Could you check a few things on this model? Use its own coordinates, in mm. A direction names the side the tool comes from. Coordinates: 2 decimals unless noted, no trailing zeros. Order: outer loops, then holes, each group sorted by start corner. A loop starts at its lowest first (then second) coordinate and runs counter-clockwise, first axis right, second up. Notation, with made-up numbers: (35, 1.25) - (41, 1.25) arc R16 cw to (41, 8.25) - close; hole circle Ø2 at (56, 66.25). An arc over 180 degrees is marked (long way). Answer as CSV lines item,"result". Start each with the question number.
1. I want a section at B-B, the plane z = -3.7. List the corners of the cut face in (x, y) for me, and give its area (3 significant figures).
2. I need wall thicknesses on probe 1 along X at (y, z) = (-1.8, -0.3); probe 2 along X at (y, z) = (-0.35, -0.1). Which ranges of each line are inside material? Lowest first, please.
3. For faces 1 (the face through (2, -0.5, 0)), 2 (the face through (-1, -0.5, -4)), 3 (the face through (0.5, 0, -2)), which set-ups out of +Z, -Z, +X, -X, +Y, -Y let a thin tool reach every point of the face, with its end or its side?
4. I want a section at C-C, the plane x = 1. List the corners of the cut face in (y, z) for me.
5. For pin 1 (1.1 mm diameter, centred on x = 2.5, y = 0, fed in from -Z); pin 2 (1 mm diameter, centred on y = 0, z = -1.5, fed in from +X); pin 3 (0.5 mm diameter, centred on x = 1.5, z = 0, fed in from -Y), each with a flat end and sliding along its axis, tell me the tip position at first contact or that it passes through.
from build123d import *

# Parameters (mm, degrees)
PAD_DEPTH    = 0.5
PAD001_DEPTH = 0.5
PAD002_DEPTH = 0.5
PAD003_DEPTH = 0.5
SKETCH004_W  = 0.8
SKETCH004_H  = 0.15
SKETCH006_W  = 0.8
SKETCH006_H  = 0.15


with BuildPart() as part:
    # Sketch → Pad (new body, symmetric)
    with BuildSketch(Plane.XY):
        Polygon((0.5, 0.5), (4.5, 0.5), (4.5, -0.5), (0.5, -0.5), (-0.5, -0.5), (-0.5, 0.5), align=None)
    extrude(amount=PAD_DEPTH, both=True)

    # Sketch001 → Pad001 (join, symmetric)
    with BuildSketch(Plane.YZ):
        Polygon((-0.5, 0.5), (0.5, 0.5), (0.5, -0.5), (0.5, -4.5), (-0.5, -4.5), (-0.5, -0.5), align=None)
    extrude(amount=PAD001_DEPTH, both=True)

    # Sketch002 (on DatumPlane) → Pad002 (join, symmetric)
    with BuildSketch(Plane.XY.offset(-4)):
        Polygon((-4.5, 0.5), (-0.5, 0.5), (0.5, 0.5), (0.5, -0.5), (-0.5, -0.5), (-4.5, -0.5), align=None)
    extrude(amount=PAD002_DEPTH, both=True)

    # Sketch003 → Pad003 (join, symmetric)
    with BuildSketch(Plane.XY):
        Polygon((-0.5, 0.5), (0.5, 0.5), (0.5, -0.5), (0.5, -2.5), (-0.5, -2.5), (-0.5, -0.5), align=None)
    extrude(amount=PAD003_DEPTH, both=True)

    # Sketch004 → Revolution (revolve)
    with BuildSketch(Plane.XY):
        with Locations((4.9, 0.075)):
            Rectangle(SKETCH004_W, SKETCH004_H)
    revolve(axis=Axis((0, 0, 0), (-1, 0, 0)))

    # Sketch005 → Revolution001 (revolve)
    with BuildSketch(Plane.XY):
        with BuildLine():
            ThreePointArc((5.8, 0), (5.3, 0.5), (4.8, 0))
            Line((4.8, 0), (5.3, 0))
            Line((5.3, 0), (5.8, 0))
        make_face()
    revolve(axis=Axis((0, 0, 0), (1, 0, 0)))

    # Sketch006 (on DatumPlane) → Revolution002 (revolve)
    with BuildSketch(Plane.XY.offset(-4)):
        with Locations((-4.9, 0.075)):
            Rectangle(SKETCH006_W, SKETCH006_H)
    revolve(axis=Axis((0, 0, -4), (1, 0, 0)))

    # Sketch007 (on DatumPlane) → Revolution003 (revolve)
    with BuildSketch(Plane.XY.offset(-4)):
        with BuildLine():
            ThreePointArc((-5.8, 0), (-5.3, -0.5), (-4.8, 0))
            Line((-5.3, 0), (-4.8, 0))
            Line((-5.8, 0), (-5.3, 0))
        make_face()
    revolve(axis=Axis((0, 0, -4), (1, 0, 0)))


solid = part.part
Solved:
1,outline,"circle Ø0.8 at (-5.3, 0); (-4.5, -0.5) - (0.5, -0.5) - (0.5, 0.5) - (-4.5, 0.5) - close"
1,area,"5.50 mm2"
2,probe 1,"x = -0.5 to 0.5"
2,probe 2,"x = -0.5 to 4.5, 4.96 to 5.64"
3,face 1,"+Z, -Z, +X, -Y"
3,face 2,"-Z, +X, -X, -Y"
3,face 3,"-Z, +X, +Y, -Y"
4,outline,"(-0.5, -0.5) - (0.5, -0.5) - (0.5, 0.5) - (-0.5, 0.5) - close"
5,pin 1,"stops at z = -0.5"
5,pin 2,"stops at x = 0.5"
5,pin 3,"stops at y = -0.5"
